Print and shaded views of the part. All mm, measured from the part's lowest x, y and z. Round coordinates to 2 decimals unless told otherwise and drop trailing zeros. Write each loop counter-clockwise with the first axis right and the second up, starting at its lowest first coordinate (ties: lowest second). Pieces come first, ordered by that corner, then holes. Notation, with made-up numbers: M 56.25,10 L 96.25,10 A10 ccw 96.25,27 Z; hole C 6.25,54.25 d2. An arc over 180 degrees is marked long. Write item = value, one per line.
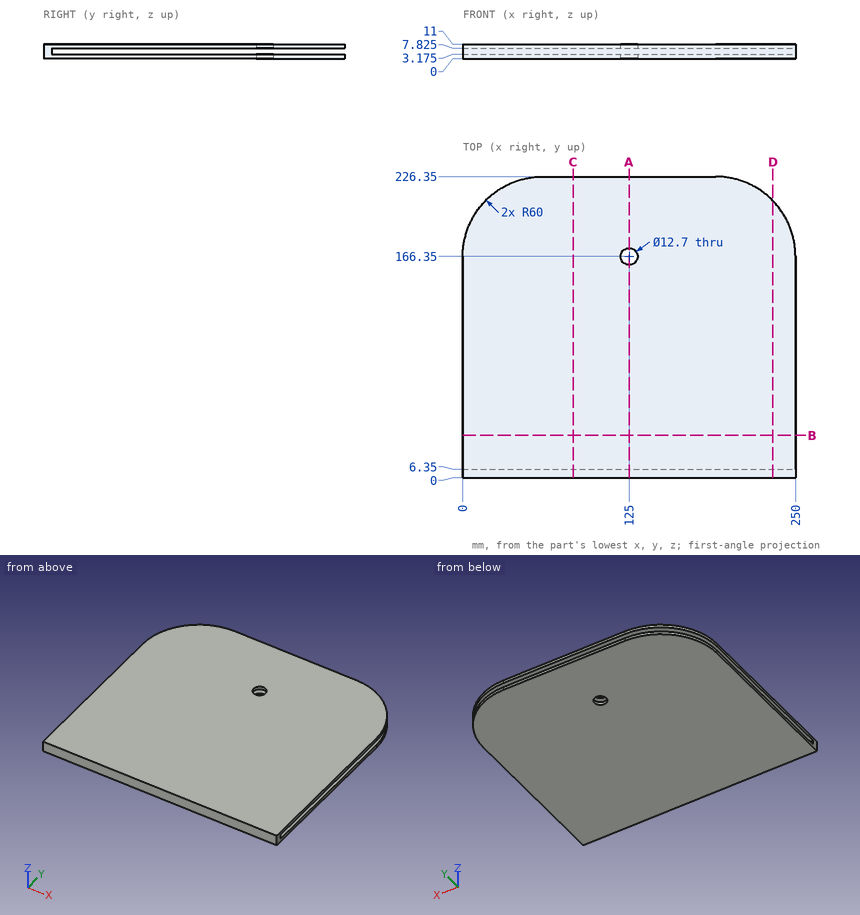
1. Band-saw the part on D-D (x = 233). List the corners of the cut face in (y, z) (3 decimals).
Responses:
outline = M 0,0 L 208.195,0 L 208.195,3.175 L 6.35,3.175 L 6.35,7.825 L 208.195,7.825 L 208.195,11 L 0,11 Z
2. Band-saw the part on C-C (x = 83). List the corners of the cut face in (y, z) (3 decimals), plus the area to 3 significant figures.
Responses:
outline = M 0,0 L 226.35,0 L 226.35,3.175 L 6.35,3.175 L 6.35,7.825 L 226.35,7.825 L 226.35,11 L 0,11 Z
area = 1,470 mm²
3. Band-saw the part on B-B (y = 32). List the corners of the cut face in (x, z) (3 decimals).
Responses:
outline = M 0,0 L 250,0 L 250,3.175 L 0,3.175 Z; M 0,7.825 L 250,7.825 L 250,11 L 0,11 Z
4. Probe probe 1 along Z at (x, y) = (184.5, 157.5) (3 decimals); probe 2 along Y at (x, z) = (125, 9.05); probe 3 along Y at (x, z) = (215, 4.5). List the from-to ranges inside material, lowest first.
Responses:
probe_1 = 0 to 3.175, 7.825 to 11
probe_2 = 0 to 160, 172.7 to 226.35
probe_3 = 0 to 6.35
5. Band-saw the part on A-A (x = 125). List the corners of the cut face in (y, z) (3 decimals).
Responses:
outline = M 0,0 L 160,0 L 160,3.175 L 6.35,3.175 L 6.35,7.825 L 160,7.825 L 160,11 L 0,11 Z; M 172.7,0 L 226.35,0 L 226.35,3.175 L 172.7,3.175 Z; M 172.7,7.825 L 226.35,7.825 L 226.35,11 L 172.7,11 Z
6. Flat gauge pins, fed straight in: pin 1 (4 mm diameter, centred on y = 171, z = 1, fed in from +X); pin 2 (1.4 mm diameter, centred on x = 104, z = 6, fed in from +Y). Where does each tip first touch, or does it go through?
Responses:
pin_1 = 249.94
pin_2 = 6.35
